Work out the finished part from the listing and answer in its coordinate system (mm). Face numbers are marked on the shaded views. A direction names the side the tool comes from. Give positions to 0.01 mm unless a question says otherwise; leave off trailing zeros. Write each loop counter-clockwise with the first axis right and the second up, starting at its lowest first coordinate (ties: lowest second). Pieces come first, ordered by that corner, then holes.
1) A tool of negligible diameter and unlimited length cuts with its end or side. For the marked faces 1, 2 and 3, from which of +Z, -Z, +X, -X, +Y, -Y can it reach the whole face along a straight path? Write none if from no direction.
2) Given pin 1 Ø3 at (x, y) = (-4, 35) entering from -Z, flat-ended and moving along its own axis, determine where the tip first touches the part or whether it passes through.
3) Find section A-A (z = 0.8). Determine the outline of the cut face in (x, y).
4) Determine the mould class of the marked faces 4, 5 and 6 for opening direction X: pulls with the +X half, pulls with the -X half, needs draft (parallel to the pull), parting line crosses it, or undercut.
5) Find section B-B (y = 25.5). Determine the outline of the cut face in (x, z).
6) Find section C-C (x = 16). Determine the outline of the cut face in (y, z), plus the area to 3 significant figures.
7) Straight lines are drawn through the part: probe 1 along X at (y, z) = (24, 2.6); probe 2 along Y at (x, z) = (12, 1.55); probe 3 along X at (y, z) = (10, 2.05). For each, find the intervals that lie inside material, in ascending order.
8) Find section D-D (x = -7). Determine the outline of the cut face in (y, z), plus the area to 3 significant figures.
```python
from build123d import *

# Parameters (mm, degrees)
F1_DEPTH = 3
F2_D     = 5.8
F2_DEPTH = 3
F2_TIP   = 1.7424957952


with BuildPart() as f1:
    # F0 (on Top) → F1 (new body)
    with BuildSketch(Plane.XY):
        with BuildLine():
            ThreePointArc((2.4641827419, 32.7869937197), (1.2508461254, 32.4804226982), (0, 32.5198626147))
            Line((0, 32.5198626147), (0, 18.7683064789))
            Line((0, 18.7683064789), (2.0859143711, 29.4431521909))
            Line((2.0859143711, 29.4431521909), (17.7015492515, 19.1490593441))
            Line((17.7015492515, 19.1490593441), (13.9597342261, 0))
            Line((13.9597342261, 0), (0, 0))
            Line((0, 0), (0, -10.5885749888))
            Line((0, -10.5885749888), (21.2067912519, -10.5885749888))
            Line((21.2067912519, -10.5885749888), (26.5765645376, 16.8917003894))
            Line((26.5765645376, 16.8917003894), (2.4641827419, 32.7869937197))
        make_face()
        with BuildLine():
            Line((0, 18.7683064789), (0, 32.5198626147))
            ThreePointArc((0, 32.5198626147), (-0.178141111, 32.5543418855), (-0.3547474317, 32.5959746011))
            Line((-0.3547474317, 32.5959746011), (-8.7932087481, -10.5885749888))
            Line((-8.7932087481, -10.5885749888), (0, -10.5885749888))
            Line((0, -10.5885749888), (0, 0))
            Line((0, 0), (-3.6674141493, 0))
            Line((-3.6674141493, 0), (0, 18.7683064789))
        make_face()
        with BuildLine():
            Line((-0.3547474317, 32.5959746011), (0, 34.4114250112))
            Line((0, 34.4114250112), (2.4641827419, 32.7869937197))
            ThreePointArc((2.4641827419, 32.7869937197), (4.5003263885, 34.443479167), (5.2658624981, 36.9542120184))
            ThreePointArc((5.2658624981, 36.9542120184), (-1.9916051188, 40.510385853), (-0.3547474317, 32.5959746011))
        make_face()
        with BuildLine():
            Line((2.4641827419, 32.7869937197), (0, 34.4114250112))
            Line((0, 34.4114250112), (0, 32.5198626147))
            ThreePointArc((0, 32.5198626147), (1.2508461254, 32.4804226982), (2.4641827419, 32.7869937197))
        make_face()
        with BuildLine():
            Line((0, 32.5198626147), (0, 34.4114250112))
            Line((0, 34.4114250112), (-0.3547474317, 32.5959746011))
            ThreePointArc((-0.3547474317, 32.5959746011), (-0.178141111, 32.5543418855), (0, 32.5198626147))
        make_face()
    extrude(amount=F1_DEPTH)

    # F2
    with Locations(Plane(origin=(0, 0, 0), x_dir=(1, 0, 0), z_dir=(0, 0, -1))):
        with Locations((0.7658624981, -36.9542120184)):
            Hole(F2_D / 2, depth=F2_DEPTH)
            with Locations((0, 0, -(F2_DEPTH + F2_TIP / 2))):  # 118° drill point
                Cone(0, F2_D / 2, F2_TIP, mode=Mode.SUBTRACT)


solid = f1.part
```
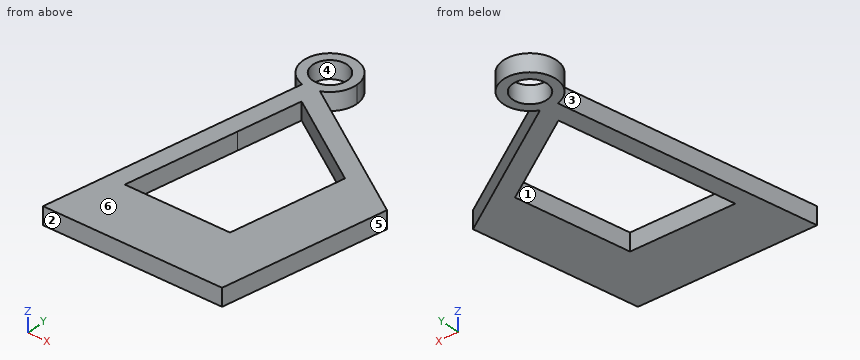
Results:
1. face 1: +Z, -Z
1. face 2: +Z, -Z, +X, -X, -Y
1. face 3: +Z, -Z, -X
2. pin 1: stops at z = 0
3. outline: (-8.79, -10.59) - (21.21, -10.59) - (26.58, 16.89) - (2.46, 32.79) arc R4.5 ccw (long way) to (-0.35, 32.6) - close; hole (-3.67, 0) - (13.96, 0) - (17.7, 19.15) - (2.09, 29.44) - close; hole circle Ø5.8 at (0.77, 36.95)
4. face 4: undercut
4. face 5: pulls with the +X half
4. face 6: needs draft
5. outline: (-1.74, 0) - (1.32, 0) - (1.32, 3) - (-1.74, 3) - close; (8.07, 0) - (13.52, 0) - (13.52, 3) - (8.07, 3) - close
6. outline: (-10.59, 0) - (10.44, 0) - (10.44, 3) - (-10.59, 3) - close; (20.27, 0) - (23.86, 0) - (23.86, 3) - (20.27, 3) - close
6. area: 73.9 mm2
7. probe 1: x = -2.03 to 1.02, 10.34 to 15.79
7. probe 2: y = -10.59 to 0, 22.91 to 26.5
7. probe 3: x = -4.77 to -1.71, 15.91 to 25.23
8. outline: (-10.59, 0) - (-1.41, 0) - (-1.41, 3) - (-10.59, 3) - close
8. area: 27.5 mm2
